```python
from build123d import *

# Parameters (mm, degrees)
BOSS_EXTRUDE1_START  = -17
BOSS_EXTRUDE1_DEPTH  = 34
SKETCH2_R            = 14.3
CUT_EXTRUDE1_DEPTH   = 32
SKETCH3_R            = 7.975
CUT_EXTRUDE2_DEPTH   = 68.982497748
SKETCH4_R            = 12.5
CUT_EXTRUDE3_DEPTH   = 69.946500999
FILLET5_R            = 10
FILLET6_R            = 10
FILLET5_OF_MIRROR1_R = 10
FILLET6_OF_MIRROR1_R = 10
SKETCH12_W           = 71.004828568
SKETCH12_H           = 128.011080482
CUT_EXTRUDE4_DEPTH   = 25
SKETCH13_W           = 23.55
SKETCH13_H           = 45.2
CUT_EXTRUDE5_DEPTH   = 2
CUT_EXTRUDE6_DEPTH   = 5
SKETCH15_R           = 12.5
SKETCH15_R_2         = 7.975
BOSS_EXTRUDE2_DEPTH  = 5
FILLET7_R            = 1
FILLET8_R            = 1


with BuildPart() as part:
    # Sketch1 → Boss-Extrude1 (new body)
    with BuildSketch(Plane.YZ.offset(BOSS_EXTRUDE1_START)):
        with BuildLine():
            Line((-14.9, 0), (-14.9, 58.1))
            Line((-14.9, 58.1), (14.9, 58.1))
            Line((14.9, 58.1), (14.9, 0))
            ThreePointArc((14.9, 0), (0, -14.9), (-14.9, 0))
        make_face()
    boss_extrude1 = extrude(amount=BOSS_EXTRUDE1_DEPTH)

    # Sketch2 → Cut-Extrude1 (cut)
    with BuildSketch(Plane.YZ.offset(17)):
        with Locations(Location((0, 0, 0), (0, 0, 270))):
            Circle(SKETCH2_R)
    cut_extrude1 = extrude(amount=-CUT_EXTRUDE1_DEPTH, mode=Mode.SUBTRACT)

    # Sketch3 → Cut-Extrude2 (cut, through all)
    with BuildSketch(Plane.YZ.offset(-15)):
        with Locations(Location((0, 0, 0), (0, 0, 270))):
            Circle(SKETCH3_R)
    cut_extrude2 = extrude(amount=-CUT_EXTRUDE2_DEPTH, mode=Mode.SUBTRACT)

    # Sketch4 → Cut-Extrude3 (cut, through all)
    with BuildSketch(Plane.YZ.offset(17)):
        with Locations(Location((0, 35.8, 0), (0, 0, 270))):
            Circle(SKETCH4_R)
    cut_extrude3 = extrude(amount=-CUT_EXTRUDE3_DEPTH, mode=Mode.SUBTRACT)

    # Fillet5
    fillet5_edges = [part.edges().sort_by_distance(p)[0] for p in [
        (0, 14.9, 58.1),
    ]]
    fillet(fillet5_edges, radius=FILLET5_R)

    # Fillet6
    fillet6_edges = [part.edges().sort_by_distance(p)[0] for p in [
        (0, -14.9, 58.1),
    ]]
    fillet(fillet6_edges, radius=FILLET6_R)

    # Mirror1: Boss-Extrude1, Cut-Extrude1, Cut-Extrude2, Cut-Extrude3 across plane
    add(boss_extrude1.mirror(Plane.XY))
    add(cut_extrude1.mirror(Plane.XY), mode=Mode.SUBTRACT)
    add(cut_extrude2.mirror(Plane.XY), mode=Mode.SUBTRACT)
    add(cut_extrude3.mirror(Plane.XY), mode=Mode.SUBTRACT)

    # Fillet5 of Mirror1
    fillet5_of_mirror1_edges = [part.edges().sort_by_distance(p)[0] for p in [
        (0, 14.9, -58.1),
    ]]
    fillet(fillet5_of_mirror1_edges, radius=FILLET5_OF_MIRROR1_R)

    # Fillet6 of Mirror1
    fillet6_of_mirror1_edges = [part.edges().sort_by_distance(p)[0] for p in [
        (0, -14.9, -58.1),
    ]]
    fillet(fillet6_of_mirror1_edges, radius=FILLET6_OF_MIRROR1_R)

    # Sketch12 → Cut-Extrude4 (cut)
    with BuildSketch(Plane.YZ.offset(17)):
        Rectangle(SKETCH12_W, SKETCH12_H)
    extrude(amount=-CUT_EXTRUDE4_DEPTH, mode=Mode.SUBTRACT)

    # Sketch13 → Cut-Extrude5 (cut)
    with BuildSketch(Plane.YZ.offset(-8)):
        with Locations((3.125, 0)):
            Rectangle(SKETCH13_W, SKETCH13_H)
    extrude(amount=-CUT_EXTRUDE5_DEPTH, mode=Mode.SUBTRACT)

    # Sketch14 → Cut-Extrude6 (cut)
    with BuildSketch(Plane.YZ.offset(-10)):
        with BuildLine():
            Line((-6.1496227, -22.630710053), (-3.65, -22.6))
            Line((-3.65, -22.6), (0, -22.6))
            Line((0, -22.6), (0, -14.3))
            ThreePointArc((0, -14.3), (-1.840302956, -14.181088993), (-3.65, -13.82633357))
            ThreePointArc((-3.65, -13.82633357), (-4.983735764, -13.403446491), (-6.269759745, -12.852241545))
            Line((-6.269759745, -12.852241545), (-6.1496227, -22.630710053))
        make_face()
    cut_extrude6 = extrude(amount=-CUT_EXTRUDE6_DEPTH, mode=Mode.SUBTRACT)

    # Mirror2: Cut-Extrude6 across plane
    add(cut_extrude6.mirror(Plane.XY), mode=Mode.SUBTRACT)

    # Sketch15 → Boss-Extrude2 (add)
    with BuildSketch(Plane(origin=(-17, 0, 0), x_dir=(0, -1, 0), z_dir=(-1, 0, 0))):
        with BuildLine():
            Line((-4.9, -58.1), (4.9, -58.1))
            ThreePointArc((4.9, -58.1), (11.971067812, -55.171067812), (14.9, -48.1))
            Line((14.9, -48.1), (14.9, 48.1))
            ThreePointArc((14.9, 48.1), (11.971067812, 55.171067812), (4.9, 58.1))
            Line((4.9, 58.1), (-4.9, 58.1))
            ThreePointArc((-4.9, 58.1), (-11.971067812, 55.171067812), (-14.9, 48.1))
            Line((-14.9, 48.1), (-14.9, -48.1))
            ThreePointArc((-14.9, -48.1), (-11.971067812, -55.171067812), (-4.9, -58.1))
        make_face()
        with Locations(Location((0, 35.95, 0), (0, 0, 180.34377674))):
            Circle(SKETCH15_R, mode=Mode.SUBTRACT)
        with Locations(Location((0, 0, 0), (0, 0, 90))):
            Circle(SKETCH15_R_2, mode=Mode.SUBTRACT)
        with Locations(Location((0, -35.8, 0), (0, 0, 90))):
            Circle(SKETCH15_R, mode=Mode.SUBTRACT)
    extrude(amount=BOSS_EXTRUDE2_DEPTH)

    # Fillet7
    fillet7_edges = [part.edges().sort_by_distance(p)[0] for p in [
        (-10, 0, -18.45),
    ]]
    fillet(fillet7_edges, radius=FILLET7_R)

    # Fillet8
    fillet8_edges = [part.edges().sort_by_distance(p)[0] for p in [
        (-10, 0, 18.45),
    ]]
    fillet(fillet8_edges, radius=FILLET8_R)


solid = part.part
```
Geometry check sheet. Reference: the model listing, model coordinates, mm. A direction names the side the tool comes from. Coordinates: 2 decimals unless noted, no trailing zeros. Order: outer loops, then holes, each group sorted by start corner. A loop starts at its lowest first (then second) coordinate and runs counter-clockwise, first axis right, second up.
Q1. Tool access check on faces 4 (the face through (-14.9, 8.45, -45.01)), 5 (the face through (-12.44, 8.45, 45.01)), 6 (the face through (-19.465, -1.702, 23.566)), 7 (the face through (-22, -10, 1)), 8 (the face through (-10, -7, 17)). Record the directions out of +Z, -Z, +X, -X, +Y, -Y that give a thin tool (end or side, any length) a straight path to the whole face; none if there is none.
Reply:
face 4: +X, -X
face 5: +X
face 6: -X
face 7: +Z, -Z, -X, +Y, -Y
face 8: +X, +Y
Q2. Thickness scan on probe 1 along Z at (x, y) = (-9.5, -7); probe 2 along Y at (x, z) = (-10.75, -35.8); probe 3 along Z at (x, y) = (-10, -10). Record the ranges inside material, lowest first.
Reply:
probe 1: z = -57.88 to -46.16, -25.44 to -22.6, 22.6 to 25.44, 46.16 to 57.88
probe 2: y = -14.9 to -12.5, 12.5 to 14.9
probe 3: z = -56.7 to -43.3, -28.3 to -10.22, 10.22 to 28.3, 43.3 to 56.7
Q3. Sectioned sample at C-C on y = -9.75. Record the cut outline in (x, z), and give its area (3 significant figures).
Reply:
outline: (-22, -56.85) - (-8, -56.85) - (-8, -43.62) - (-22, -43.62) - close; (-22, -27.98) - (-8, -27.98) - (-8, -10.46) - (-15, -10.46) - (-15, 10.46) - (-8, 10.46) - (-8, 27.98) - (-17, 27.98) - (-17, 28.13) - (-22, 28.13) - close; (-22, 43.77) - (-17, 43.77) - (-17, 43.62) - (-8, 43.62) - (-8, 56.85) - (-22, 56.85) - close
area: 1,010 mm2
Q4. Sectioned sample at D-D on y = -1.25. Record the cut outline in (x, z).
Reply:
outline: (-22, -58.1) - (-8, -58.1) - (-8, -48.24) - (-22, -48.24) - close; (-22, -23.36) - (-8, -23.36) - (-8, -22.6) - (-15, -22.6) - (-15, -7.88) - (-22, -7.88) - close; (-22, 7.88) - (-15, 7.88) - (-15, 22.6) - (-8, 22.6) - (-8, 23.36) - (-17, 23.36) - (-17, 23.51) - (-22, 23.51) - close; (-22, 48.39) - (-17, 48.39) - (-17, 48.24) - (-8, 48.24) - (-8, 58.1) - (-22, 58.1) - close
Q5. Sectioned sample at A-A on x = -16. Record the cut outline in (y, z) (3 decimals).
Reply:
outline: (-14.9, -48.1) arc R10 ccw to (-4.9, -58.1) - (4.9, -58.1) arc R10 ccw to (14.9, -48.1) - (14.9, 48.1) arc R10 ccw to (4.9, 58.1) - (-4.9, 58.1) arc R10 ccw to (-14.9, 48.1) - close; hole circle Ø25 at (0, -35.8); hole circle Ø25 at (0, 35.8); hole circle Ø15.95 at (0, 0)
Q6. Draft check along Z on faces 1 (the face through (-13, 0, 19)), 2 (the face through (-8, -10, -12)), 3 (the face through (-9, 3, 22.6)). Enter one of: released by +Z, released by -Z, zero draft, split by the parting line, or undercut.
Reply:
face 1: undercut
face 2: zero draft
face 3: undercut
Q7. Sectioned sample at B-B on z = -35.8. Record the cut outline in (x, y), and give its area (3 significant figures).
Reply:
outline: (-22, -14.9) - (-8, -14.9) - (-8, -12.5) - (-22, -12.5) - close; (-22, 12.5) - (-8, 12.5) - (-8, 14.9) - (-22, 14.9) - close
area: 67.2 mm2
Q8. Depth check by flat-ended pin: pin 1 Ø7 at (y, z) = (6.5, 2.5) entering from +X; pin 2 Ø3 at (y, z) = (-7, -19) entering from +X; pin 3 Ø1 at (x, z) = (-8.5, 18.5) entering from +Y. Enter the tip coordinate at first touch or a pass-through.
Reply:
pin 1: stops at x = -15
pin 2: stops at x = -10
pin 3: stops at y = -8.65
